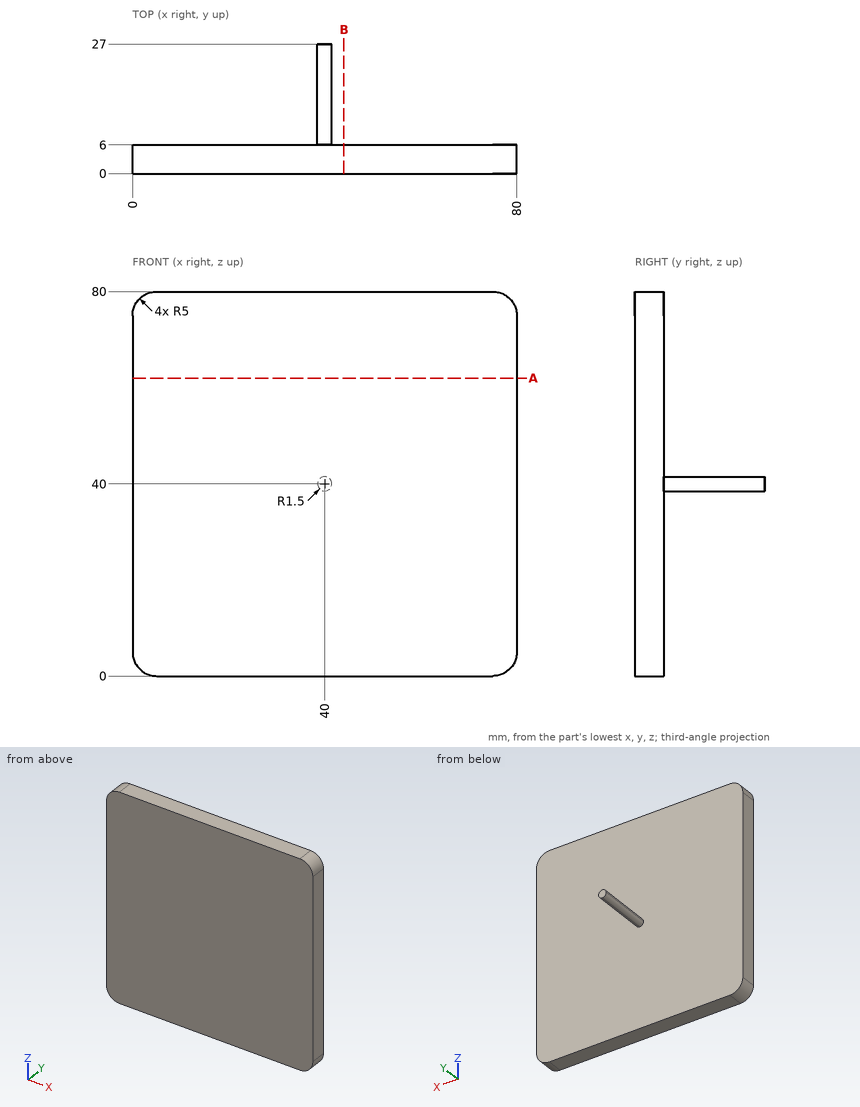
Input: dimensioned drawing with shaded views. Units: mm. Origin: part minimum x, y, z. Coordinates: 2 decimals unless noted, no trailing zeros. Loops run counter-clockwise (first coordinate to the right, second up) from the corner with the lowest first, then second, coordinate; pieces in that order, holes last. Notation, with made-up numbers: (62.5, -25) -> (69.5, -25) arc R7 cw to (69.5, -13) -> close; hole circle Ø10 at (86.25, 54). An arc over 180 degrees is marked (long way). Use a Markdown table: item, result. Add a question column.
(1) Line query: line 1 along Y through (x, z) = (70, 29.5). Output: solid intervals per line, ascending.
(2) Section query A-A, the plane z = 62. Return loops of the section in (x, y), plus the area to 3 significant figures.
(3) Section query B-B, the plane x = 44. Return loops of the section in (y, z).
(4) Pin query (flat end, axial travel): pin 1 Ø24 at (x, z) = (54.5, 42) entering from +Y; pin 2 Ø5 at (y, z) = (19, 43) entering from -X. Return the tip coordinate at first contact, or that it passes through.
Answer:
| question | item | result |
|---|---|---|
| 1 | line 1 | y = 0 to 6 |
| 2 | outline | (0, 0) -> (80, 0) -> (80, 6) -> (0, 6) -> close |
| 2 | area | 480 mm^2 |
| 3 | outline | (0, 0) -> (6, 0) -> (6, 80) -> (0, 80) -> close |
| 4 | pin 1 | stops at y = 6 |
| 4 | pin 2 | stops at x = 38.59 |
